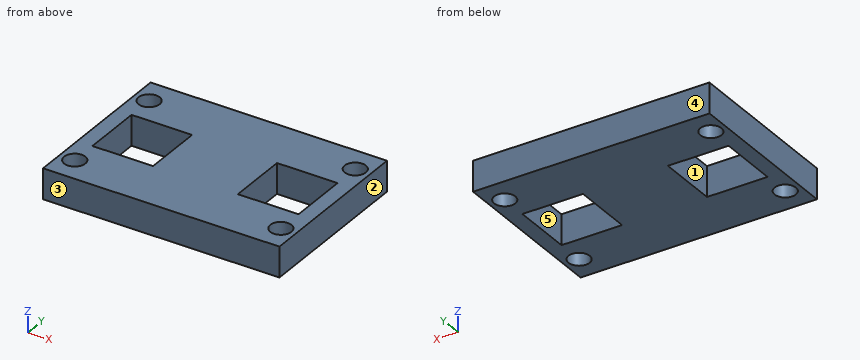
from build123d import *

# Parameters (mm, degrees)
F0_W     = 39
F0_H     = 27.55
F1_DEPTH = 5
F2_R     = 1.75
F3_DEPTH = 25
F4_W     = 10
F4_H     = 10
F5_DEPTH = 25


with BuildPart() as f1:
    # F0 (on Top) → F1 (new body)
    with BuildSketch(Plane.XY):
        Rectangle(F0_W, F0_H)
    extrude(amount=F1_DEPTH)

    # F2 (on face) → F3 (cut)
    with BuildSketch(Plane.XY.offset(5)):
        with Locations((-17, 9.525)):
            Circle(F2_R)
        with Locations((-17, -9.525)):
            Circle(F2_R)
        with Locations((17, -9.525)):
            Circle(F2_R)
        with Locations((17, 9.525)):
            Circle(F2_R)
    extrude(amount=-F3_DEPTH, mode=Mode.SUBTRACT)

    # F4 (on face) → F5 (cut)
    with BuildSketch(Plane.XY.offset(5)):
        with Locations((-12, 0)):
            Rectangle(F4_W, F4_H)
        with Locations((12, 0)):
            Rectangle(F4_W, F4_H)
    extrude(amount=-F5_DEPTH, mode=Mode.SUBTRACT)


solid = f1.part
Build history of the part. All positions in model axes, mm. Face numbers are marked on the shaded views. A direction names the side the tool comes from. Give positions to 0.01 mm unless a question says otherwise; leave off trailing zeros. Order: outer loops, then holes, each group sorted by start corner. A loop starts at its lowest first (then second) coordinate and runs counter-clockwise, first axis right, second up. Notation, with made-up numbers: M -23.75,53.25 L 9.25,53.25 A21 ccw 9.25,69.25 Z; hole C 19,43 d1. An arc over 180 degrees is marked long. Use one line per item in the form item = value.
1) Two-plate mould, pull along X, no slides. Class the marked faces 1, 2 and 3: released by +X, released by -X, zero draft, split by the parting line, or undercut.
Calculated:
face_1 = undercut
face_2 = released by +X
face_3 = zero draft
2) Saw through at D-D (z = 2.2). Give the cut face in (x, y) (3 decimals), plus the area to 3 significant figures.
Calculated:
outline = M -19.5,-13.775 L 19.5,-13.775 L 19.5,13.775 L -19.5,13.775 Z; hole C -17,-9.525 d3.5; hole C -17,9.525 d3.5; hole M -17,-5 L -7,-5 L -7,5 L -17,5 Z; hole M 7,-5 L 17,-5 L 17,5 L 7,5 Z; hole C 17,-9.525 d3.5; hole C 17,9.525 d3.5
area = 836 mm2
3) Tool access for the marked faces 4 and 5: list every direction of +Z, -Z, +X, -X, +Y, -Y with a clear straight run to the whole face (end or side of a thin tool).
Calculated:
face_4 = +Z, -Z, +X, -X, +Y
face_5 = +Z, -Z
4) Drop a flat-ended pin along its axis: pin 1 (4 mm diameter, centred on x = 17, y = 9.525, fed in from +Z). Give the stop position or say it passes through.
Calculated:
pin_1 = 5
5) Saw through at A-A (y = 0.75). Give the cut face in (x, z).
Calculated:
outline = M -19.5,0 L -17,0 L -17,5 L -19.5,5 Z; M -7,0 L 7,0 L 7,5 L -7,5 Z; M 17,0 L 19.5,0 L 19.5,5 L 17,5 Z
6) Probe probe 1 along X at (y, z) = (0.25, 1.7); probe 2 along Y at (x, z) = (-7.5, 3.25) (3 decimals); probe 3 along Y at (x, z) = (18, 4.4) (3 decimals). List the from-to ranges inside material, lowest first.
Calculated:
probe_1 = -19.5 to -17, -7 to 7, 17 to 19.5
probe_2 = -13.775 to -5, 5 to 13.775
probe_3 = -13.775 to -10.961, -8.089 to 8.089, 10.961 to 13.775
7) Saw through at B-B (x = 10). Give the cut face in (y, z) (3 decimals), plus the area to 4 significant figures.
Calculated:
outline = M -13.775,0 L -5,0 L -5,5 L -13.775,5 Z; M 5,0 L 13.775,0 L 13.775,5 L 5,5 Z
area = 87.75 mm2
8) Saw through at C-C (x = -16.5). Give the cut face in (y, z) (3 decimals), plus the area to 3 significant figures.
Calculated:
outline = M -13.775,0 L -11.202,0 L -11.202,5 L -13.775,5 Z; M -7.848,0 L -5,0 L -5,5 L -7.848,5 Z; M 5,0 L 7.848,0 L 7.848,5 L 5,5 Z; M 11.202,0 L 13.775,0 L 13.775,5 L 11.202,5 Z
area = 54.2 mm2
